from build123d import *

# Parameters (mm, degrees)
SCHIZZO1_W                   = 53
SCHIZZO1_H                   = 31.5
ESTRUSIONE_ESTRUSIONE1_DEPTH = 1.5
SCHIZZO2_R                   = 1.25
TAGLIO_ESTRUSIONE1_DEPTH     = 1.5
SCHIZZO3_R                   = 5.7
ESTRUSIONE_ESTRUSIONE2_DEPTH = 9
SCHIZZO4_W                   = 7.4
SCHIZZO4_H                   = 7.4
ESTRUSIONE_ESTRUSIONE3_DEPTH = 4


with BuildPart() as part:
    # Schizzo1 → Estrusione-Estrusione1 (new body)
    with BuildSketch(Plane(origin=(0, 0, 0), x_dir=(1, 0, 0), z_dir=(0, 1, 0))):
        Rectangle(SCHIZZO1_W, SCHIZZO1_H)
    extrude(amount=ESTRUSIONE_ESTRUSIONE1_DEPTH)

    # Schizzo2 → Taglio-Estrusione1 (cut)
    with BuildSketch(Plane(origin=(0, 1.5, 0), x_dir=(1, 0, 0), z_dir=(0, 1, 0))):
        with Locations((-21.5, 11.75)):
            Circle(SCHIZZO2_R)
        with Locations((21, 11.75)):
            Circle(SCHIZZO2_R)
        with Locations((21, -10.75)):
            Circle(SCHIZZO2_R)
        with Locations((-21.5, -10.75)):
            Circle(SCHIZZO2_R)
    extrude(amount=-TAGLIO_ESTRUSIONE1_DEPTH, mode=Mode.SUBTRACT)

    # Schizzo3 → Estrusione-Estrusione2 (add)
    with BuildSketch(Plane(origin=(0, 1.5, 0), x_dir=(1, 0, 0), z_dir=(0, 1, 0))):
        with Locations((-11.5, 1.75)):
            Circle(SCHIZZO3_R)
        with Locations((9, -8.75)):
            Circle(SCHIZZO3_R)
        with Locations((9, 9.25)):
            Circle(SCHIZZO3_R)
    extrude(amount=ESTRUSIONE_ESTRUSIONE2_DEPTH)

    # Schizzo4 → Estrusione-Estrusione3 (add)
    with BuildSketch(Plane(origin=(0, 10.5, 0), x_dir=(1, 0, 0), z_dir=(0, 1, 0))):
        with Locations((-11.5, 1.75)):
            Rectangle(SCHIZZO4_W, SCHIZZO4_H)
        with Locations((9, 9.25)):
            Rectangle(SCHIZZO4_W, SCHIZZO4_H)
        with Locations((9, -8.75)):
            Rectangle(SCHIZZO4_W, SCHIZZO4_H)
    extrude(amount=ESTRUSIONE_ESTRUSIONE3_DEPTH)


solid = part.part
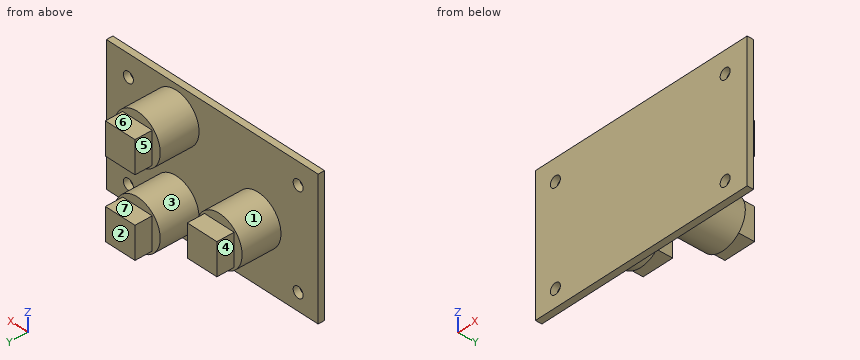
For this review, take the finished solid that the model builds, in its own axes (mm). Face numbers are marked on the shaded views. A direction names the side the tool comes from. Give positions to 0.01 mm unless a question says otherwise; leave off trailing zeros. Loops run counter-clockwise (first coordinate to the right, second up) from the corner with the lowest first, then second, coordinate; pieces in that order, holes last. Notation, with made-up numbers: M 22,77 L 75,77 A17 cw 75,98 Z; hole C 38,36 d6. An arc over 180 degrees is marked long. Answer as a JSON object with one key per item and string values. Group by question number.
Q1. Tool access review of the marked faces 5, 6 and 7: name each direction out of +Z, -Z, +X, -X, +Y, -Y from which nothing blocks a thin tool from reaching the whole face with its end or side.
Q2. For probe 1 along X at (y, z) = (1.1, -11.75); probe 2 along Z at (x, y) = (-21.5, 0.7); probe 3 along Y at (x, z) = (-0.5, 9), list the stretches that pass through material, from the lowest coordinate up. Write a range as [from, to].
Q3. Add section D-D on z = 8.75. Give the boundary of the cut face in (x, y).
Q4. Add section A-A on x = 21. Give the boundary of the cut face in (y, z), and give its area (4 significant figures).
Q5. Mouldability with a two-part tool opening along X and no side actions: class the marked faces 1, 2, 3 and 4 as +X half, -X half, draft (parallel to the pull), parting line (faces both ways), or undercut.
Q6. Add section B-B on x = -11.5. Give the boundary of the cut face in (y, z), and give its area (3 significant figures).
Q7. Insertion check: P1, Ø4.5, axis at y = 12.5, z = -1.5, coming from the -X side; P2, Ø2, axis at x = 9.5, y = 12.5, coming from the -Z side; P3, Ø3, axis at y = 12.5, z = -2.5, coming from the +X side. Each pin has a flat end and moves straight along its axis. Give the tip position at first contact, or say it passes through.
Q8. Add section C-C on y = 2.75. Give the boundary of the cut face in (x, z).
Checked values:
{
 "1": {"face 5": "+Z, -Z, -X, +Y", "face 6": "+Z, +X, -X, +Y", "face 7": "+X, -X, +Y"},
 "2": {"probe 1": "[-26.5, -22.75], [-20.25, 19.75], [22.25, 26.5]", "probe 2": "[-15.75, -13], [-10.5, 9.5], [12, 15.75]", "probe 3": "[0, 1.5]"},
 "3": {"outline": "M -26.5,0 L 26.5,0 L 26.5,1.5 L 14.7,1.5 L 14.7,10.5 L 12.7,10.5 L 12.7,14.5 L 5.3,14.5 L 5.3,10.5 L 3.3,10.5 L 3.3,1.5 L -26.5,1.5 Z"},
 "4": {"outline": "M 0,-15.75 L 1.5,-15.75 L 1.5,-13 L 0,-13 Z; M 0,-10.5 L 1.5,-10.5 L 1.5,9.5 L 0,9.5 Z; M 0,12 L 1.5,12 L 1.5,15.75 L 0,15.75 Z", "area": "39.75 mm²"},
 "5": {"face 1": "undercut", "face 2": "draft", "face 3": "undercut", "face 4": "-X half"},
 "6": {"outline": "M 0,-15.75 L 1.5,-15.75 L 1.5,-7.45 L 10.5,-7.45 L 10.5,-5.45 L 14.5,-5.45 L 14.5,1.95 L 10.5,1.95 L 10.5,3.95 L 1.5,3.95 L 1.5,15.75 L 0,15.75 Z", "area": "179 mm²"},
 "7": {"P1": "x = -17.2", "P2": "z = -12.95", "P3": "x = -7.8"},
 "8": {"outline": "C -11.5,-1.75 d11.4; C 9,-9.25 d11.4; C 9,8.75 d11.4"}
}
